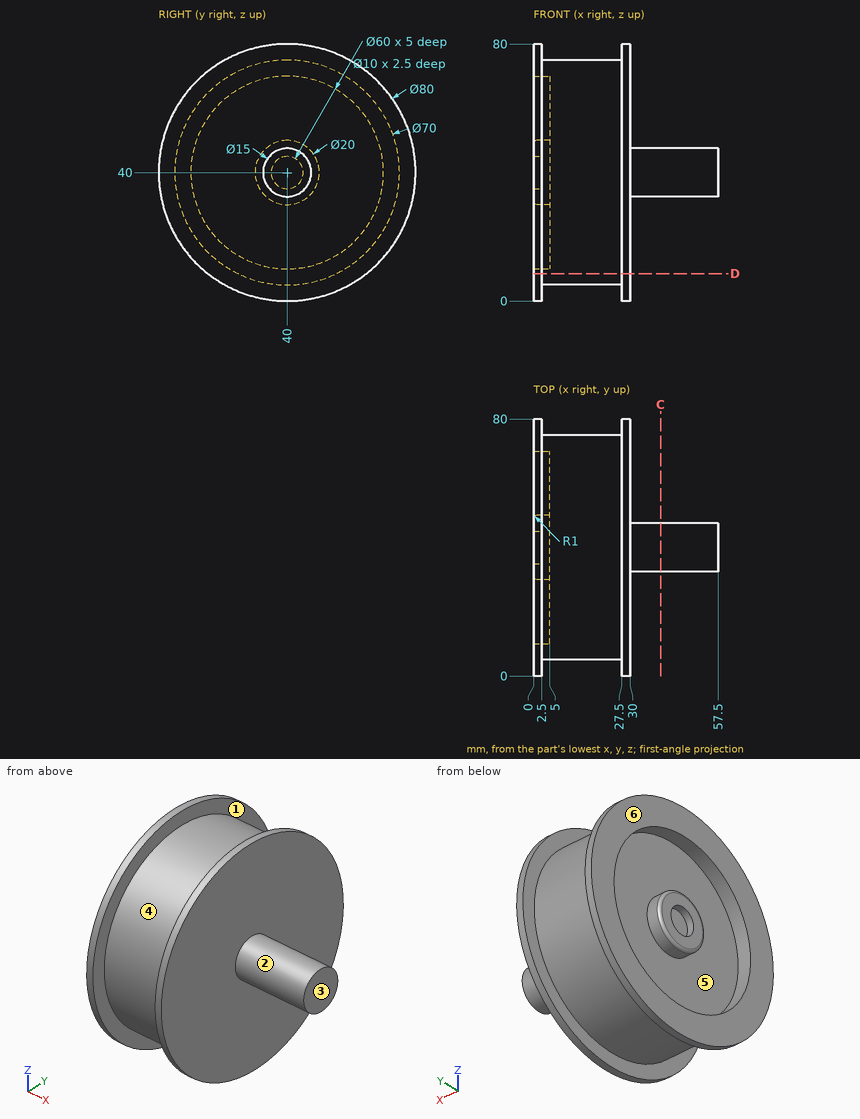
Source: three-view drawing plus pictorial views. Frame: mm from the lowest corner of the part. A direction names the side the tool comes from. Round coordinates to 2 decimals unless told otherwise and drop trailing zeros. Loops run counter-clockwise (first coordinate to the right, second up) from the corner with the lowest first, then second, coordinate; pieces in that order, holes last.
Q1. Ray query, line 1 (Y direction, x = 1, z = 40); line 2 (Y direction, x = 0.5, z = 40); line 3 (X direction, y = 14.5, z = 69). Return the intervals inside material, ascending.
Q2. First-contact query: P1, Ø8, axis at y = 56.5, z = 33.5, coming from the +X side; P2, Ø1, axis at x = 24.5, y = 11.5, coming from the -Z side; P3, Ø10, axis at x = 20, y = 38, coming from the -Z side. Flat tips, straight axial feed; report the tip coordinate or a pass-through.
Q3. Mould query, pull axis Y, two halves, no side actions, for the marked faces 4, 5 and 6. Classes: pulls with the +Y half, pulls with the -Y half, needs draft (parallel to the pull), parting line crosses it, or undercut.
Q4. Section D-D, the plane z = 8.5. Return loops of the section in (x, y), plus the area to 3 significant figures.
Q5. Access query for the marked faces 1, 2 and 3. Directions: +Z, -Z, +X, -X, +Y, -Y. A direction counts if a zero-diameter tool reaches every point of the face in a straight line with its end or side. Return the directions, or none.
Q6. Section C-C, the plane x = 39.5. Return loops of the section in (y, z).
Solutions:
1. line 1: y = 0 to 10, 30 to 35, 45 to 50, 70 to 80
1. line 2: y = 0 to 10, 30.13 to 35, 45 to 49.87, 70 to 80
1. line 3: x = 0 to 2.5, 27.5 to 30
2. P1: stops at x = 30
2. P2: stops at z = 19
2. P3: stops at z = 5
3. face 4: parting line crosses it
3. face 5: undercut
3. face 6: needs draft
4. outline: (0, 15.35) - (2.5, 15.35) - (2.5, 24.74) - (27.5, 24.74) - (27.5, 15.35) - (30, 15.35) - (30, 64.65) - (27.5, 64.65) - (27.5, 55.26) - (2.5, 55.26) - (2.5, 64.65) - (0, 64.65) - close
4. area: 1,010 mm2
5. face 1: none
5. face 2: +X
5. face 3: +Z, -Z, +X, +Y, -Y
6. outline: circle Ø15 at (40, 40)
